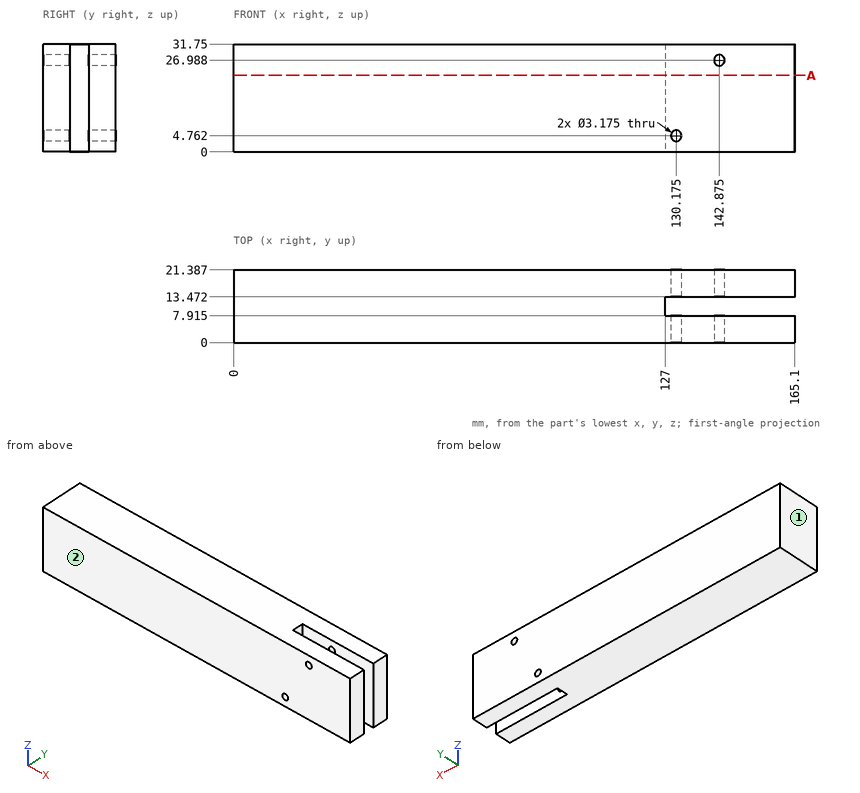
Print and shaded views of the part. All mm, measured from the part's lowest x, y and z. Coordinates: 2 decimals unless noted, no trailing zeros. Order: outer loops, then holes, each group sorted by start corner. A loop starts at its lowest first (then second) coordinate and runs counter-clockwise, first axis right, second up.
Item 1: Saw through at A-A on z = 22.5. List the corners of the cut face in (x, y) (1 decimal), then the cut area to 3 significant figures.
Filled in:
outline: (0, 0) - (165.1, 0) - (165.1, 7.9) - (127, 7.9) - (127, 13.5) - (165.1, 13.5) - (165.1, 21.4) - (0, 21.4) - close
area: 3,320 mm2
Item 2: Drill centre lines: L1, parallel to Y at x = 128.5, z = 29 (1 decimal); L2, parallel to X at y = 9.5, z = 12; L3, parallel to X at y = 16.5, z = 26.5 (1 decimal). Where is each one in solid material? Low to high.
Filled in:
L1: y = 0 to 7.9, 13.5 to 21.4
L2: x = 0 to 127
L3: x = 0 to 141.4, 144.4 to 165.1
Item 3: Mould opens along X. For the marked faces 1 and 2 say: released by +X, released by -X, zero draft, split by the parting line, or undercut.
Filled in:
face 1: released by -X
face 2: zero draft
Item 4: Drop flat-ended pins along their axis: pin 1 Ø2.5 at (x, z) = (130.18, 4.76) entering from +Y; pin 2 Ø2 at (y, z) = (11, 25.5) entering from +X. Give the stop position or say it passes through.
Filled in:
pin 1: passes through
pin 2: stops at x = 127
